Check sheet for the modelled part. Datum: model origin and axes. Units: mm. Face numbers are marked on the shaded views. A direction names the side the tool comes from. Give positions to 0.01 mm unless a question says otherwise; leave off trailing zeros. Write each loop counter-clockwise with the first axis right and the second up, starting at its lowest first coordinate (ties: lowest second). Pieces come first, ordered by that corner, then holes. Notation, with made-up numbers: (2.5, -38.75) -> (59.5, -38.75) arc R21 ccw to (59.5, -3.75) -> close; hole circle Ø4 at (37, 17.25). An arc over 180 degrees is marked (long way). Return JSON: item names as keys, results as strings.
Autodesk Inventor part; units mm, degrees
ref_plane "作業平面1" through (-10, 0, -30) normal (-1, 0, 0) x (0, 0, 1)
ref_plane "YZ Plane" through (0, 0, 0) normal (1, 0, 0) x (0, 1, 0)
ref_plane "XZ Plane" through (0, 0, 0) normal (0, 1, 0) x (-1, 0, 0)
sketch "スケッチ1" plane through (0, 0, 0) normal (0, 1, 0) x (-1, 0, 0)
  line L0 (0, 0) -> (20, 0)
  line L1 (20, 0) -> (20, -30)
  line L2 (20, -30) -> (0, -30)
  line L3 (0, -30) -> (0, 0)
  dimension "d0" = 20
  dimension "d1" = 30
extrude "押し出し1" add sketch "スケッチ1" along normal blind 24
sketch "スケッチ2" plane through (0, 0, 0) normal (1, 0, 0) x (0, 0, -1)
  line L0 (0, 0) -> (0, 24)
  line L1 (0, 16) -> (0, 24)
  line L2 (0, 24) -> (5, 24)
  line L3 (5, 24) -> (0, 16)
  dimension "d4" = 5
  dimension "d5" = 8
extrude "押し出し2" cut sketch "スケッチ2" against normal through all
sketch "スケッチ3" plane through (-20, 0, -30) normal (-1, 0, 0) x (0, 0, 1)
  circle A0 centre (22.5, 19) radius 2.5
  line L0 (30, 0) -> (30, 16)
  line L1 (0, 24) -> (25, 24)
  circle A1 centre (20, 19) radius 2.5
  line L2 (17.5, 21.5) -> (25, 21.5)
  line L3 (25, 21.5) -> (25, 16.5) construction
  line L4 (25, 16.5) -> (17.5, 16.5)
  line L5 (17.5, 16.5) -> (17.5, 21.5) construction
  point P0 (22.5, 21.5)
  point P1 (20, 21.5)
  point P2 (20, 16.5)
  point P3 (22.5, 16.5)
  dimension "d8" = 5
  dimension "d9" = 7.5
  dimension "d10" = 5
  dimension "d11" = 5
  dimension "d12" = 7.5
extrude "押し出し3" add sketch "スケッチ3" along normal blind 3
ref_plane "作業平面1" through (-10, 0, -30) normal (-1, 0, 0) x (0, 0, 1)
mirror "ミラー1" about plane through (-10, 0, -30) normal (-1, 0, 0) of "押し出し3"
sketch "スケッチ4" plane through (3, 19, -10) normal (1, 0, 0) x (0, 0, -1)
  arc A0 (-2.5, 2.5) -> (-2.5, -2.5) centre (-2.5, 0) ccw
  circle A1 centre (-2.5, 0) radius 1.25
  point P0 (-10, -19)
  dimension "d16" = 2.5
extrude "押し出し4" add sketch "スケッチ4" against normal blind 50
properties part number "Motor"
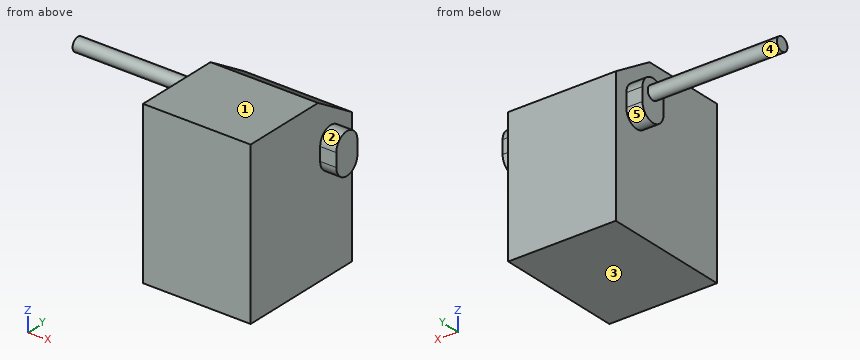
(1) Cross-section at C-C on y = 9.25. Enter the section's corners in (x, z), then the cut area to 3 significant figures.
Reply:
{"outline": "(-20, -30) -> (0, -30) -> (0, 0) -> (-20, 0) -> close", "area": "600 mm^2"}
(2) Depth check by flat-ended pin: pin 1 Ø4 at (x, z) = (-25.5, -10.5) entering from +Y; pin 2 Ø12 at (y, z) = (17, -27) entering from +X; pin 3 Ø1.2 at (x, z) = (2, -8.5) entering from +Y. Enter the tip coordinate at first touch or a pass-through.
Reply:
{"pin 1": "y = 19.75", "pin 2": "x = 0", "pin 3": "y = 21.5"}
(3) Cross-section at B-B on z = -2. Enter the section's corners in (x, y), then the cut area to 3 significant figures.
Reply:
{"outline": "(-20, 0) -> (0, 0) -> (0, 19.2) -> (-20, 19.2) -> close", "area": "384 mm^2"}
(4) Cross-section at D-D on y = 19. Enter the section's corners in (x, z) (3 decimals).
Reply:
{"outline": "(-47, -8.75) -> (-23, -8.75) -> (-23, -12.5) -> (-20, -12.5) -> (-20, -30) -> (0, -30) -> (0, -12.5) -> (3, -12.5) -> (3, -5) -> (0, -5) -> (0, -1.875) -> (-20, -1.875) -> (-20, -5) -> (-23, -5) -> (-23, -6.25) -> (-47, -6.25) -> close"}
(5) Thickness scan on L1, parallel to X at y = 20.5, z = -15; L2, parallel to Z at x = -14, y = 20.75. Record the ranges inside material, lowest first.
Reply:
{"L1": "-20 to 0", "L2": "-30 to -2.97"}
(6) Set-up check for the marked faces 1, 2, 3, 4 and 5: record each of +Z, -Z, +X, -X, +Y, -Y from which the full face is reachable in a straight line by a thin tool's end or side.
Reply:
{"face 1": "+Z, +X, -X, +Y, -Y", "face 2": "+Z, +X", "face 3": "-Z, +X, -X, +Y, -Y", "face 4": "-X", "face 5": "-Z, -X"}
(7) Cross-section at A-A on x = -6. Enter the section's corners in (y, z).
Reply:
{"outline": "(0, -30) -> (24, -30) -> (24, -5) -> (16, 0) -> (0, 0) -> close"}
